from build123d import *

# Parameters (mm, degrees)
EXTRUDE_1_DEPTH     = 355
CUT_EXTRUDE_1_DEPTH = 146
SKETCH_3_R          = 5
CUT_EXTRUDE_2_DEPTH = 10


with BuildPart() as part:
    # Эскиз1 → Вытянуть-Тонкостенный1 (new body)
    with BuildSketch(Plane(origin=(0, 0, 0), x_dir=(0, 0, -1), z_dir=(1, 0, 0))):
        Polygon((0, 0), (0, 87), (145, 87), (145, 0), (142, 0), (142, 84), (3, 84), (3, 0), align=None)
    extrude(amount=EXTRUDE_1_DEPTH)

    # Эскиз2 → Вырез-Вытянуть1 (cut, through all)
    with BuildSketch(Plane.XY):
        with BuildLine():
            Line((0, 65.12405332), (0, 0))
            Line((0, 0), (350.278484056, 0))
            add(Edge.make_bspline(
                [(0, 65.12405332), (7.933841156, 41.786887325), (88.835587811, 42.671964813), (115.548592719, -4.570720396), (275.808566843, 2.451761606), (350.278484056, 0)],
                knots=[0, 0, 0, 0, 0.332901295, 0.537301133, 1, 1, 1, 1], degree=3))
        make_face()
    extrude(amount=-CUT_EXTRUDE_1_DEPTH, mode=Mode.SUBTRACT)

    # Эскиз3 → Вырез-Вытянуть2 (cut)
    with BuildSketch(Plane(origin=(0, 87, 0), x_dir=(1, 0, 0), z_dir=(0, 1, 0))):
        with Locations((322, 117.5)):
            Circle(SKETCH_3_R)
        with Locations((212, 117.5)):
            Circle(SKETCH_3_R)
        with Locations((102, 117.5)):
            Circle(SKETCH_3_R)
        with Locations((212, 27.5)):
            Circle(SKETCH_3_R)
        with Locations((102, 27.5)):
            Circle(SKETCH_3_R)
        with Locations((322, 27.5)):
            Circle(SKETCH_3_R)
    extrude(amount=-CUT_EXTRUDE_2_DEPTH, mode=Mode.SUBTRACT)


solid = part.part
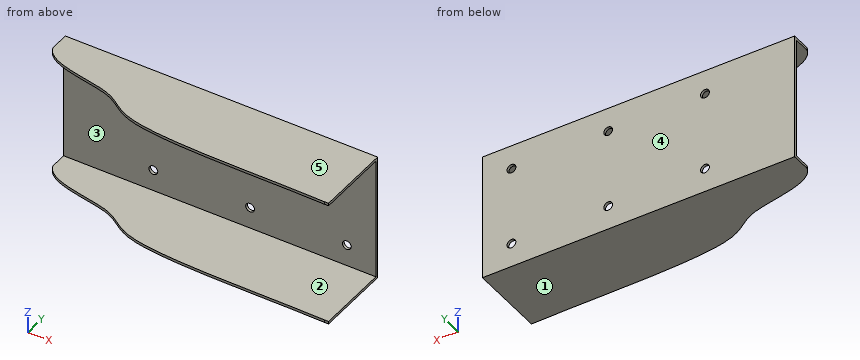
Verification items for the finished model (mm, model axes). Face numbers are marked on the shaded views. A direction names the side the tool comes from. Round coordinates to 2 decimals unless told otherwise and drop trailing zeros. Loops run counter-clockwise (first coordinate to the right, second up) from the corner with the lowest first, then second, coordinate; pieces in that order, holes last. Notation, with made-up numbers: (-12.5, 40.5) - (18.5, 40.5) arc R10 ccw to (18.5, 52.5) - close; hole circle Ø2 at (14, 5). An arc over 180 degrees is marked (long way). Write item = value, one per line.
Q1. Tool access check on the marked faces 1 and 2. Record the directions out of +Z, -Z, +X, -X, +Y, -Y that give a thin tool (end or side, any length) a straight path to the whole face; none if there is none.
Here are the results:
face_1 = -Z, +X, -X, +Y, -Y
face_2 = +X, -X, -Y
Q2. Sectioned sample at C-C on z = -83.5. Record the boundary of the cut face in (x, y).
Here are the results:
outline = (0, 84) - (355, 84) - (355, 87) - (0, 87) - close
Q3. Sectioned sample at B-B on x = 212. State how many separate pieces and enclosed holes the cut face has, plus the area to 3 significant figures.
Here are the results:
separate_pieces = 3
enclosed_holes = 0
area = 869 mm^2
Q4. Sectioned sample at A-A on z = -27.5. Record the boundary of the cut face in (x, y).
Here are the results:
outline = (0, 84) - (97, 84) - (97, 87) - (0, 87) - close; (107, 84) - (207, 84) - (207, 87) - (107, 87) - close; (217, 84) - (317, 84) - (317, 87) - (217, 87) - close; (327, 84) - (355, 84) - (355, 87) - (327, 87) - close
Q5. Mould release check, pull along Z, two halves, no side actions. Record for the marked faces 3, 4 and 5: +Z half, -Z half, draft (parallel to the pull), parting line (faces both ways), or undercut.
Here are the results:
face_3 = undercut
face_4 = draft
face_5 = +Z half
Q6. Depth check by flat-ended pin: pin 1 (13 mm diameter, centred on x = 102, z = -117.5, fed in from -Y). Enter the tip coordinate at first touch or a pass-through.
Here are the results:
pin_1 = 84
Q7. Material ranges on L1, parallel to Z at x = 212, y = 84.75; L2, parallel to X at y = 84.85, z = -27.5; L3, parallel to Z at x = 203, y = 81, recorded low to high.
Here are the results:
L1 = -145 to -122.5, -112.5 to -32.5, -22.5 to 0
L2 = 0 to 97, 107 to 207, 217 to 317, 327 to 355
L3 = -145 to -142, -3 to 0
